The drawing under review shows one solid part. Ordinate dimensions are in mm from its lowest x, y, z. A direction names the side the tool comes from. Round coordinates to 2 decimals unless told otherwise and drop trailing zeros. Write each loop counter-clockwise with the first axis right and the second up, starting at its lowest first coordinate (ties: lowest second). Pieces come first, ordered by that corner, then holes. Notation, with made-up numbers: (0.5, 1.25) -> (34.5, 1.25) arc R22 ccw to (34.5, 35.25) -> close; hole circle Ø4 at (-38, -18.5). An arc over 180 degrees is marked (long way). Write item = value, one per line. Start each with the question number.
Item 1: Add section B-B, the plane y = 4.55. State the section outline as (x, z) points (1 decimal).
Item 2: For pin 1 Ø0.6 at (x, z) = (3.5, 1.5) entering from -Y; pin 2 Ø0.9 at (y, z) = (2.5, 11) entering from -X; pin 3 Ø0.6 at (y, z) = (3, 1.5) entering from +X, all flat-tipped, find the tip position at first contact; note any pin that passes through.
Item 3: To check wall thickness, follow L1, parallel to Z at x = 3, y = 3.55 (1 decimal); L2, parallel to X at y = 2.2, z = 6.5 (1 decimal); L3, parallel to Y at x = 0.5, z = 12.25. State the ranges of each line that lie inside material, in increasing order.
Item 4: Mouldability with a two-part tool opening along Z and no side actions: class the marked faces 3, 4 and 5 as released by +Z, released by -Z, zero draft, split by the parting line, or undercut.
Item 5: Add section C-C, the plane y = 2.7. State the section outline as (x, z) points (1 decimal).
Item 6: Machinability: for the marked faces 1 and 2, which of the approach directions +Z, -Z, +X, -X, +Y, -Y give a long, thin tool a straight path to every point of the face, cutting with its end or side? Answer none if there is none.
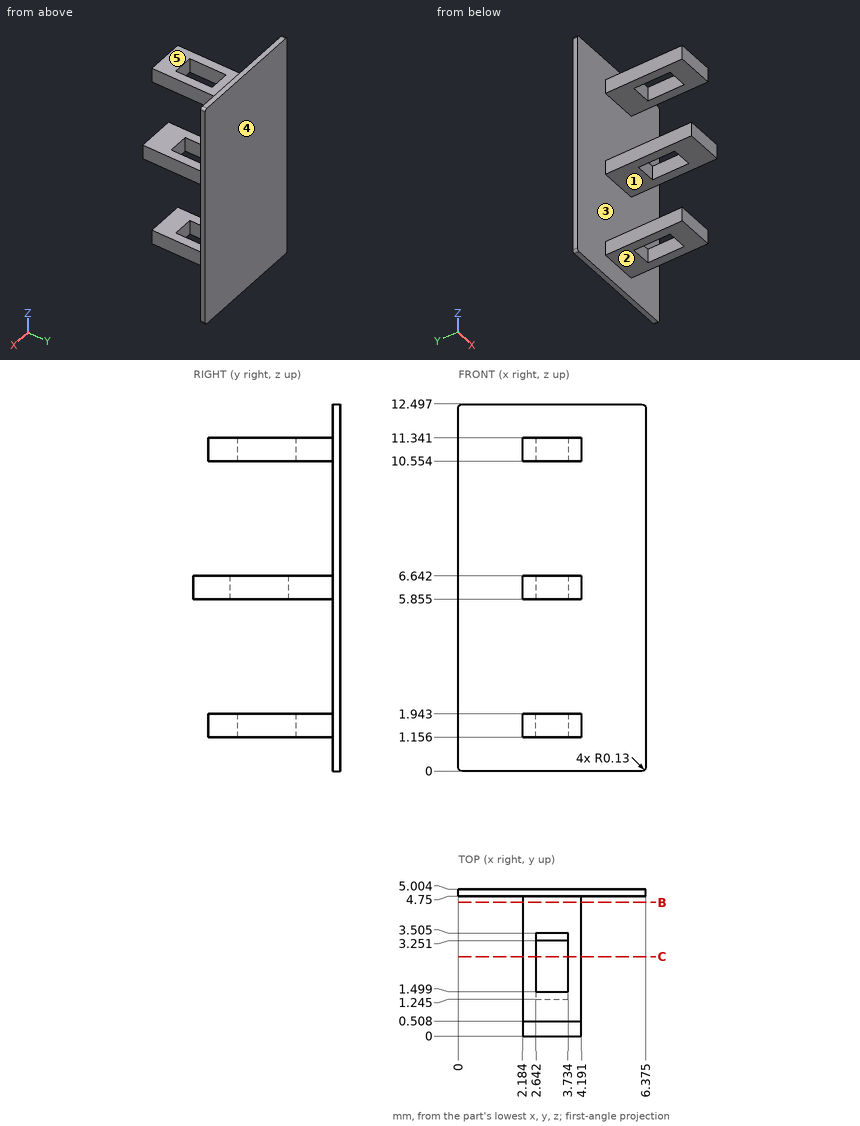
Result set:
q1.outline = (2.2, 1.2) -> (4.2, 1.2) -> (4.2, 1.9) -> (2.2, 1.9) -> close; (2.2, 5.9) -> (4.2, 5.9) -> (4.2, 6.6) -> (2.2, 6.6) -> close; (2.2, 10.6) -> (4.2, 10.6) -> (4.2, 11.3) -> (2.2, 11.3) -> close
q2.pin_1 = 0.51
q2.pin_2 = 2.18
q2.pin_3 = 4.19
q3.L1 = 1.2 to 1.9, 5.9 to 6.6, 10.6 to 11.3
q3.L2 = 2.2 to 2.6, 3.7 to 4.2
q3.L3 = 4.75 to 5
q4.face_3 = undercut
q4.face_4 = zero draft
q4.face_5 = released by +Z
q5.outline = (2.2, 1.2) -> (2.6, 1.2) -> (2.6, 1.9) -> (2.2, 1.9) -> close; (2.2, 5.9) -> (2.6, 5.9) -> (2.6, 6.6) -> (2.2, 6.6) -> close; (2.2, 10.6) -> (2.6, 10.6) -> (2.6, 11.3) -> (2.2, 11.3) -> close; (3.7, 1.2) -> (4.2, 1.2) -> (4.2, 1.9) -> (3.7, 1.9) -> close; (3.7, 5.9) -> (4.2, 5.9) -> (4.2, 6.6) -> (3.7, 6.6) -> close; (3.7, 10.6) -> (4.2, 10.6) -> (4.2, 11.3) -> (3.7, 11.3) -> close
q6.face_1 = +X, -X, -Y
q6.face_2 = -Z, +X, -X, -Y
